```python
from build123d import *

# Parameters (mm, degrees)
SKETCH1_W            = 100
SKETCH1_H            = 100
SKETCH1_W_2          = 92
SKETCH1_H_2          = 92
BOSS_EXTRUDE1_DEPTH  = 40
BOSS_EXTRUDE2_DEPTH  = 2
M2_CLEARANCE_HOLE1_D = 2.4


with BuildPart() as part:
    # Sketch1 → Boss-Extrude1 (new body)
    with BuildSketch(Plane(origin=(0, 0, 0), x_dir=(1, 0, 0), z_dir=(0, 1, 0))):
        Rectangle(SKETCH1_W, SKETCH1_H)
        Rectangle(SKETCH1_W_2, SKETCH1_H_2, mode=Mode.SUBTRACT)
    extrude(amount=BOSS_EXTRUDE1_DEPTH)

    # Sketch2 → Boss-Extrude2 (add)
    with BuildSketch(Plane(origin=(0, 0, 0), x_dir=(-1, 0, 0), z_dir=(0, -1, 0))):
        with BuildLine():
            Line((-46, 32), (-46, 46))
            Line((-46, 46), (-32, 46))
            ThreePointArc((-32, 46), (-36.100505063, 36.100505063), (-46, 32))
        make_face()
        with BuildLine():
            Line((32, 46), (46, 46))
            Line((46, 46), (46, 32))
            ThreePointArc((46, 32), (36.100505063, 36.100505063), (32, 46))
        make_face()
        with BuildLine():
            Line((46, -32), (46, -46))
            Line((46, -46), (32, -46))
            ThreePointArc((32, -46), (36.100505063, -36.100505063), (46, -32))
        make_face()
        with BuildLine():
            Line((-32, -46), (-46, -46))
            Line((-46, -46), (-46, -32))
            ThreePointArc((-46, -32), (-36.100505063, -36.100505063), (-32, -46))
        make_face()
    extrude(amount=-BOSS_EXTRUDE2_DEPTH)

    # M2 Clearance Hole1 (through all)
    with Locations(Plane(origin=(40, 0, 40), x_dir=(0, 0, -1), z_dir=(0, -1, 0))):
        with Locations((0, 0), (80, 0), (80, -80), (0, -80)):
            Hole(M2_CLEARANCE_HOLE1_D / 2)


solid = part.part
```
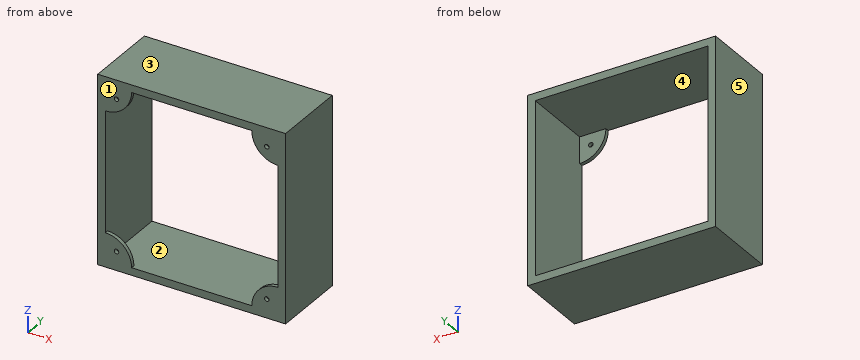
The model under review builds one solid part; all positions refer to its coordinate system, in mm. Face numbers are marked on the shaded views. A direction names the side the tool comes from. Round coordinates to 2 decimals unless told otherwise and drop trailing zeros. Loops run counter-clockwise (first coordinate to the right, second up) from the corner with the lowest first, then second, coordinate; pieces in that order, holes last. Notation, with made-up numbers: (50, 78.5) -> (105, 78.5) arc R33 cw to (105, 117.5) -> close; hole circle Ø7 at (-17, 52.5). An arc over 180 degrees is marked (long way). Answer as a JSON object with one key per item and string values. Group by question number.
1) We need section C-C on y = 20. Write out the cut boundary in (x, z).
2) For line 1 (X direction, y = 19, z = 23.5); line 2 (X direction, y = 1.05, z = -40), list the stretches that pass through material, from the lowest coordinate up. Write a range as [from, to].
3) For the marked faces 1 and 2, list the 3-axis set-ups (+Z, -Z, +X, -X, +Y, -Y) from which the entire face can be reached by the end or side of a thin tool; tool diameter is ignored.
4) We need section B-B on x = 24. Write out the cut boundary in (y, z), then the cut area to 3 significant figures.
5) We need section D-D on z = -40. Write out the cut boundary in (x, y).
6) For pin 1 Ø2 at (x, z) = (40, 40) entering from -Y; pin 2 Ø7 at (x, z) = (38, 38.5) entering from +Y, all flat-tipped, find the tip position at first contact; note any pin that passes through.
7) Mouldability with a two-part tool opening along X and no side actions: class the marked faces 3, 4 and 5 as released by +X, released by -X, zero draft, split by the parting line, or undercut.
8) We need section A-A on z = -22. Write out the cut boundary in (x, y), then the cut area to 3 significant figures.
Result set:
{
 "1": {"outline": "(-50, -50) -> (50, -50) -> (50, 50) -> (-50, 50) -> close; hole (-46, -46) -> (46, -46) -> (46, 46) -> (-46, 46) -> close"},
 "2": {"line 1": "[-50, -46], [46, 50]", "line 2": "[-50, -41.2], [-38.8, -33.35], [33.35, 38.8], [41.2, 50]"},
 "3": {"face 1": "+Z, -Z, +X, -X, -Y", "face 2": "+Y"},
 "4": {"outline": "(0, -50) -> (40, -50) -> (40, -46) -> (0, -46) -> close; (0, 46) -> (40, 46) -> (40, 50) -> (0, 50) -> close", "area": "320 mm²"},
 "5": {"outline": "(-50, 0) -> (-41.2, 0) -> (-41.2, 2) -> (-46, 2) -> (-46, 40) -> (-50, 40) -> close; (-38.8, 0) -> (-33.35, 0) -> (-33.35, 2) -> (-38.8, 2) -> close; (33.35, 0) -> (38.8, 0) -> (38.8, 2) -> (33.35, 2) -> close; (41.2, 0) -> (50, 0) -> (50, 40) -> (46, 40) -> (46, 2) -> (41.2, 2) -> close"},
 "6": {"pin 1": "through", "pin 2": "y = 2"},
 "7": {"face 3": "zero draft", "face 4": "undercut", "face 5": "released by -X"},
 "8": {"outline": "(-50, 0) -> (-46, 0) -> (-46, 40) -> (-50, 40) -> close; (46, 0) -> (50, 0) -> (50, 40) -> (46, 40) -> close", "area": "320 mm²"}
}
